Autodesk Inventor part; units mm, degrees
ref_plane "YZ Plane" through (0, 0, 0) normal (1, 0, 0) x (0, 1, 0)
ref_plane "XZ Plane" through (0, 0, 0) normal (0, 1, 0) x (-1, 0, 0)
ref_plane "XY Plane" through (0, 0, 0) normal (0, 0, 1) x (1, 0, 0)
sketch "Sketch5" plane through (0, 0, 0) normal (0, 0, 1) x (1, 0, 0)
  line L0 (52.8, -15.6) -> (52.8, -10.6)
  line L1 (52.8, -10.6) -> (49.8, -10.6)
  line L2 (49.8, -10.6) -> (49.8, -12.55)
  line L3 (44, -12.55) -> (44, -3.05)
  line L4 (49.8, -3.05) -> (49.8, -5)
  line L5 (49.8, -5) -> (52.8, -5)
  line L6 (52.8, -5) -> (52.8, 0)
  line L7 (52.8, 0) -> (7.8, 0)
  line L8 (44, -3.05) -> (49.8, -3.05)
  line L9 (44, -12.55) -> (49.8, -12.55)
  line L10 (52.8, -15.6) -> (7.8, -15.6)
  arc A0 (7.8, 0) -> (7.8, -15.6) centre (7.8, -7.8) ccw
  point P0 (0, 0)
  dimension "d41" = 5.8
  dimension "d48" = 44
  dimension "d63" = 45
  dimension "d67" = 15.6
  dimension "d71" = 0
  dimension "d72" = 36.2
  dimension "d85" = 5.6
  dimension "d86" = 9.5
  dimension "d87" = 3
extrude "Extrusion2" add sketch "Sketch5" along normal blind 12
sketch "Sketch9" plane through (0, 0, 12) normal (0, 0, 1) x (1, 0, 0)
  line L0 (52.8, 0) -> (7.8, 0)
  line L1 (7.6933, 0) -> (9.4034, -4.6985)
  line L2 (9.4034, -4.6985) -> (0.0065, -8.1187)
  arc A0 (7.8, 0) -> (7.8, -15.6) centre (7.8, -7.8) ccw
  point P0 (0, 0)
  point P1 (7.6936, -0.0007)
  dimension "d89" = 5
  dimension "d92" = 110
  dimension "d93" = 10
extrude "Extrusion6" cut sketch "Sketch9" along normal blind 8 from surface at -12
sketch "Sketch11" plane through (0, 0, 12) normal (0, 0, 1) x (1, 0, 0)
  line L0 (1.7497, 0.249) -> (7.6768, -16.0354)
  line L1 (7.6768, -16.0354) -> (-2.2601, -19.6521)
  line L2 (-2.2601, -19.6521) -> (-8.1871, -3.3677)
  line L3 (-8.1871, -3.3677) -> (1.7497, 0.249)
  line L4 (7.6936, -0.0007) -> (9.4034, -4.6985)
  point P0 (0, 0)
  dimension "d98" = 5.5
extrude "Extrusion8" cut sketch "Sketch11" against normal through all
fillet "Fillet2" radius 15 1 edges at (7.5164, -15.5948, 6)
sketch "Sketch12" plane through (0, 0, 12) normal (0, 0, 1) x (1, 0, 0)
  point P0 (0, 0)
equation "\"l1\" = 8"
properties part number "Finray_test_8_Kerbe_20deg_V4_links"
Verification items for the finished model (mm, model axes). A direction names the side the tool comes from. Coordinates: 2 decimals unless noted, no trailing zeros. Loops run counter-clockwise (first coordinate to the right, second up) from the corner with the lowest first, then second, coordinate; pieces in that order, holes last. Notation, with made-up numbers: (-4, -26.5) -> (6, -26.5) arc R22 cw to (6, 0.5) -> close; hole circle Ø10 at (34, 77.5). An arc over 180 degrees is marked (long way). Answer in a Markdown table with one row per item. Add a question column.
1. Draft check along Y on faces 1 (the face through (3.24, -3.84, 10.03)), 2 (the face through (8.536, -2.316, 3.944)), 3 (the face through (31, 0, 6)). Enter one of: +Y half, -Y half, draft (parallel to the pull), parting line (faces both ways), or undercut.
2. Depth check by flat-ended pin: P1, Ø0.6, axis at y = -12, z = 9, coming from the -X side; P2, Ø3.5, axis at x = 6.5, y = -2, coming from the -Z side; P3, Ø2, axis at y = -13.5, z = 4.5, coming from the -X side. Enter the tip coordinate at first touch or a pass-through.
3. Section check C-C, the plane y = -2.5. Enter the section's corners in (x, z).
4. Section check A-A, the plane x = 47. Enter the section's corners in (y, z), then the cut area to 3 significant figures.
5. Material ranges on probe 1 along Y at (x, z) = (48.5, 8.25); probe 2 along Z at (x, y) = (6, -3); probe 3 along X at (y, z) = (-2.75, 7.25), recorded low to high. Write a range as [from, to].
6. Access from +Z, -Z, +X, -X, +Y, -Y to the whole of each face (thin tool, end or side, straight path). Record for faces 4 (the face through (51, -10.6, 6)), 5 (the face through (6.87, -5.62, 3.94)), 6 (the face through (44, -8, 6)).
7. Section check D-D, the plane z = 2.5. Enter the section's corners in (x, y).
8. Section check B-B, the plane z = 11. Enter the section's corners in (x, y).
Derived:
| question | item | result |
|---|---|---|
| 1 | face 1 | -Y half |
| 1 | face 2 | undercut |
| 1 | face 3 | +Y half |
| 2 | P1 | stops at x = 7.93 |
| 2 | P2 | stops at z = 8 |
| 2 | P3 | stops at x = 8.89 |
| 3 | outline | (2.75, 8) -> (8.6, 8) -> (8.6, 0) -> (52.8, 0) -> (52.8, 12) -> (2.75, 12) -> close |
| 4 | outline | (-15.6, 0) -> (-12.55, 0) -> (-12.55, 12) -> (-15.6, 12) -> close; (-3.05, 0) -> (0, 0) -> (0, 12) -> (-3.05, 12) -> close |
| 4 | area | 73.2 mm² |
| 5 | probe 1 | y = [-15.6, -12.55], [-3.05, 0] |
| 5 | probe 2 | z = [8, 12] |
| 5 | probe 3 | x = [8.69, 52.8] |
| 6 | face 4 | +Z, -Z, +X |
| 6 | face 5 | -Z, -X |
| 6 | face 6 | +Z, -Z |
| 7 | outline | (4.26, -6.57) arc R15 ccw to (18.02, -15.6) -> (52.8, -15.6) -> (52.8, -10.6) -> (49.8, -10.6) -> (49.8, -12.55) -> (44, -12.55) -> (44, -3.05) -> (49.8, -3.05) -> (49.8, -5) -> (52.8, -5) -> (52.8, 0) -> (7.8, 0) arc R7.8 ccw to (7.69, 0) -> (9.4, -4.7) -> close |
| 8 | outline | (2.57, -2.01) -> (3.93, -5.73) arc R15 ccw to (18.02, -15.6) -> (52.8, -15.6) -> (52.8, -10.6) -> (49.8, -10.6) -> (49.8, -12.55) -> (44, -12.55) -> (44, -3.05) -> (49.8, -3.05) -> (49.8, -5) -> (52.8, -5) -> (52.8, 0) -> (7.8, 0) arc R7.8 ccw to start |
